The listing builds one solid part. Answer for the finished solid, in the listing's coordinates (mm). A direction names the side the tool comes from. Coordinates: 2 decimals unless noted, no trailing zeros. Order: outer loops, then holes, each group sorted by start corner. A loop starts at its lowest first (then second) coordinate and runs counter-clockwise, first axis right, second up. Notation, with made-up numbers: (67.25, 42) -> (109.25, 42) arc R16 cw to (109.25, 73) -> close; hole circle Ø7 at (9, -8.5). An arc over 180 degrees is marked (long way). Return JSON: item names as keys, results as strings.
```python
from build123d import *

# Parameters (mm, degrees)
PAD_DEPTH       = 6
PAD001_DEPTH    = 2.2
PAD002_DEPTH    = 1
PAD003_DEPTH    = 1
SKETCH004_W     = 6
SKETCH004_H     = 6
PAD004_DEPTH    = 3
SKETCH005_W     = 2.5
SKETCH005_H     = 1.5
POCKET_DEPTH    = 6.001
SKETCH006_W     = 1.5
SKETCH006_H     = 2.5
POCKET001_DEPTH = 7.001


with BuildPart() as part:
    # Sketch → Pad (new body)
    with BuildSketch(Plane.XY):
        with BuildLine():
            Line((-4, 0), (4, 0))
            ThreePointArc((-4, 0), (0, -4), (4, 0))
        make_face()
    extrude(amount=PAD_DEPTH)

    # Sketch001 (on Face1 of Pad) → Pad001 (join)
    with BuildSketch(Plane(origin=(0, 0, 0), x_dir=(-1, 0, 0), z_dir=(0, 1, 0))):
        with BuildLine():
            Line((-3, 3), (-3, 0))
            Line((-3, 0), (0, 0))
            ThreePointArc((0, 0), (2.12132, 0.87868), (3, 3))
            Line((3, 3), (3, 6))
            Line((3, 6), (0, 6))
            ThreePointArc((0, 6), (-2.12132, 5.12132), (-3, 3))
        make_face()
    extrude(amount=PAD001_DEPTH)

    # Sketch002 (on Face7 of Pad001) → Pad002 (join)
    with BuildSketch(Plane.YZ.offset(3)):
        Polygon((0, 0), (0, 6), (0.3, 0), align=None)
    extrude(amount=PAD002_DEPTH)

    # Sketch003 (on Face3 of Pad002) → Pad003 (join)
    with BuildSketch(Plane(origin=(-3, 0, 0), x_dir=(0, -1, 0), z_dir=(-1, 0, 0))):
        Polygon((0, 0), (0, 6), (-0.3, 6), align=None)
    extrude(amount=PAD003_DEPTH)

    # Sketch004 (on Face6 of Pad003) → Pad004 (join)
    with BuildSketch(Plane(origin=(0, 2.2, 0), x_dir=(-1, 0, 0), z_dir=(0, 1, 0))):
        with Locations((0, 3)):
            Rectangle(SKETCH004_W, SKETCH004_H)
    extrude(amount=PAD004_DEPTH)

    # Sketch005 (on Face18 of Pad004) → Pocket (cut, through all)
    with BuildSketch(Plane.XY.offset(6)):
        with Locations((0, 3.15)):
            Rectangle(SKETCH005_W, SKETCH005_H)
    extrude(amount=-POCKET_DEPTH, mode=Mode.SUBTRACT)

    # Sketch006 (on Face5 of Pocket) → Pocket001 (cut, through all)
    with BuildSketch(Plane.YZ.offset(3)):
        with Locations((3.15, 3)):
            Rectangle(SKETCH006_W, SKETCH006_H)
    extrude(amount=-POCKET001_DEPTH, mode=Mode.SUBTRACT)


solid = part.part
```
Item 1: The part is cut by section A-A on y = 3. Determine the outline of the cut face in (x, z).
Answer list:
{"outline": "(-3, 0) -> (-1.25, 0) -> (-1.25, 1.75) -> (-3, 1.75) -> close; (-3, 4.25) -> (-1.25, 4.25) -> (-1.25, 6) -> (-3, 6) -> close; (1.25, 0) -> (3, 0) -> (3, 1.75) -> (1.25, 1.75) -> close; (1.25, 4.25) -> (3, 4.25) -> (3, 6) -> (1.25, 6) -> close"}
Item 2: The part is cut by section B-B on z = 2.5. Determine the outline of the cut face in (x, y) (3 decimals), plus the area to 3 significant figures.
Answer list:
{"outline": "(-4, 0) arc R4 ccw to (4, 0) -> (4, 0.175) -> (3, 0.175) -> (3, 2.4) -> (-3, 2.4) -> (-3, 2.2) -> (-2.958, 2.2) -> (-2.958, 0) -> (-3, 0) -> (-3, 0.125) -> (-4, 0.125) -> close; (-3, 3.9) -> (3, 3.9) -> (3, 5.2) -> (-3, 5.2) -> close", "area": "47.5 mm2"}
Item 3: Flat-ended cylindrical pins translate along their axes: pin 1 (1.5 mm diameter, centred on y = 3.5, z = 2, fed in from -X); pin 2 (1.5 mm diameter, centred on x = 2, z = 4, fed in from -Y); pin 3 (2.5 mm diameter, centred on y = 2.5, z = 4, fed in from +X). Find the tip coordinate at first contact, or state that the pin passes through.
Answer list:
{"pin 1": "x = -3", "pin 2": "y = -3.8", "pin 3": "x = 3"}
Item 4: Determine the mould class of faces 5 (the cylindrical face through (0, -4, 3)), 6 (the flat face through (0.1, -0.5, 0)), 7 (the flat face through (0, 3.9, 3)) for opening direction X: pulls with the +X half, pulls with the -X half, needs draft (parallel to the pull), parting line crosses it, or undercut.
Answer list:
{"face 5": "parting line crosses it", "face 6": "needs draft", "face 7": "undercut"}
Item 5: The part is cut by section C-C on x = 0.5. Determine the outline of the cut face in (y, z).
Answer list:
{"outline": "(-3.97, 0) -> (2.4, 0) -> (2.4, 6) -> (2.2, 6) -> (2.2, 5.96) -> (0, 5.96) -> (0, 6) -> (-3.97, 6) -> close; (3.9, 0) -> (5.2, 0) -> (5.2, 6) -> (3.9, 6) -> close"}
Item 6: Find the intervals of material crossed by probe 1 along Y at (x, z) = (0, 2.75); probe 2 along Z at (x, y) = (-2.25, 3.5); probe 3 along Y at (x, z) = (2.5, 5), in increasing order.
Answer list:
{"probe 1": "-4 to 2.4, 3.9 to 5.2", "probe 2": "0 to 1.75, 4.25 to 6", "probe 3": "-3.12 to 0, 2.2 to 5.2"}
Item 7: The part is cut by section D-D on z = 1.5. Determine the outline of the cut face in (x, y) (3 decimals).
Answer list:
{"outline": "(-4, 0) arc R4 ccw to (4, 0) -> (4, 0.225) -> (3, 0.225) -> (3, 5.2) -> (-3, 5.2) -> (-3, 2.2) -> (-2.598, 2.2) -> (-2.598, 0) -> (-3, 0) -> (-3, 0.075) -> (-4, 0.075) -> close; hole (-1.25, 2.4) -> (1.25, 2.4) -> (1.25, 3.9) -> (-1.25, 3.9) -> close"}
Item 8: Which of the six approach directions +Z, -Z, +X, -X, +Y, -Y give full straight-line access (tool end or side, diameter ignored) to faces 1 (the flat face through (2, 3, 4.25)), 2 (the flat face through (0, 2.4, 3)), 3 (the flat face through (-2.4, 2.2, 0.6)), 4 (the flat face through (2.4, 2.2, 5.3))?
Answer list:
{"face 1": "+X, -X", "face 2": "none", "face 3": "-Z, -X", "face 4": "+Z, +X"}
